```python
from build123d import *

# Parameters (mm, degrees)
F0_W     = 22.098
F0_H     = 47.498
F1_DEPTH = 1016
F2_R     = 3.96875
F3_DEPTH = 1.651
F4_R     = 9.525
F5_DEPTH = 1.651


with BuildPart() as f1:
    # F0 (on Front) → F1 (new body)
    with BuildSketch(Plane.XZ):
        with BuildLine():
            ThreePointArc((0, 1.651), (0.483567, 0.483567), (1.651, 0))
            Line((1.651, 0), (23.749, 0))
            ThreePointArc((23.749, 0), (24.916433, 0.483567), (25.4, 1.651))
            Line((25.4, 1.651), (25.4, 49.149))
            ThreePointArc((25.4, 49.149), (24.916433, 50.316433), (23.749, 50.8))
            Line((23.749, 50.8), (1.651, 50.8))
            ThreePointArc((1.651, 50.8), (0.483567, 50.316433), (0, 49.149))
            Line((0, 49.149), (0, 1.651))
        make_face()
        with Locations((12.7, 25.4)):
            Rectangle(F0_W, F0_H, mode=Mode.SUBTRACT)
    extrude(amount=F1_DEPTH)

    # F2 (on face) → F3 (cut, through all)
    with BuildSketch(Plane.YZ.offset(25.4)):
        with Locations((-508, 25.4)):
            Circle(F2_R)
        with Locations((-53.975, 25.4)):
            Circle(F2_R)
        with Locations((-962.025, 25.4)):
            Circle(F2_R)
    extrude(amount=-F3_DEPTH, mode=Mode.SUBTRACT)

    # F4 (on face) → F5 (cut, through all)
    with BuildSketch(Plane(origin=(0, 0, 0), x_dir=(0, -1, 0), z_dir=(-1, 0, 0))):
        with Locations((508, 25.4)):
            Circle(F4_R)
        with Locations((53.975, 25.4)):
            Circle(F4_R)
        with Locations((962.025, 25.4)):
            Circle(F4_R)
    extrude(amount=-F5_DEPTH, mode=Mode.SUBTRACT)


solid = f1.part
```
The model under review builds one solid part; all positions refer to its coordinate system, in mm. A direction names the side the tool comes from. Give positions to 0.01 mm unless a question says otherwise; leave off trailing zeros. Write each loop counter-clockwise with the first axis right and the second up, starting at its lowest first coordinate (ties: lowest second). Pieces come first, ordered by that corner, then holes. Notation, with made-up numbers: (84.5, 75.25) -> (132.5, 75.25) arc R25 cw to (132.5, 103.25) -> close; hole circle Ø6 at (65.25, 44). An arc over 180 degrees is marked (long way). Answer in a Markdown table with one row per item.
1) Add section B-B on y = -292. State the section outline as (x, z) points.
Worked answers:
| item | result |
|---|---|
| outline | (0, 1.65) arc R1.65 ccw to (1.65, 0) -> (23.75, 0) arc R1.65 ccw to (25.4, 1.65) -> (25.4, 49.15) arc R1.65 ccw to (23.75, 50.8) -> (1.65, 50.8) arc R1.65 ccw to (0, 49.15) -> close; hole (1.65, 1.65) -> (23.75, 1.65) -> (23.75, 49.15) -> (1.65, 49.15) -> close |
2) Clearance check with flat-ended pins moving along their axes: P1, Ø12.5, axis at y = -508, z = 25.4, coming from the -X side; P2, Ø12, axis at x = 13.5, z = 28, coming from the +Y side. State where each tip first meets the part, or that it passes through.
Worked answers:
| item | result |
|---|---|
| P1 | x = 23.75 |
| P2 | through |
3) Tool access review of faces 4 (the flat face through (13, -501, 50.8)), 5 (the cylindrical face through (0.814, -498.484, 25.819)), 6 (the flat face through (13, -501, 1.651)): name each direction out of +Z, -Z, +X, -X, +Y, -Y from which nothing blocks a thin tool from reaching the whole face with its end or side.
Worked answers:
| item | result |
|---|---|
| face 4 | +Z, +X, -X, +Y, -Y |
| face 5 | -X |
| face 6 | +Y, -Y |
4) For L1, parallel to Z at x = 16.5, y = -584; L2, parallel to X at y = -144, z = 6.5; L3, parallel to Z at x = 1.2, y = -508 (3 decimals), list the stretches that pass through material, from the lowest coordinate up. Write a range as [from, to].
Worked answers:
| item | result |
|---|---|
| L1 | [0, 1.65], [49.15, 50.8] |
| L2 | [0, 1.65], [23.75, 25.4] |
| L3 | [0.063, 15.875], [34.925, 50.737] |
5) Add section A-A on x = 14.5. State the section outline as (y, z) points.
Worked answers:
| item | result |
|---|---|
| outline | (-1016, 0) -> (0, 0) -> (0, 1.65) -> (-1016, 1.65) -> close; (-1016, 49.15) -> (0, 49.15) -> (0, 50.8) -> (-1016, 50.8) -> close |
6) Mouldability with a two-part tool opening along Y and no side actions: class faces 1 (the flat face through (1, -1016, 27)), 2 (the flat face through (25.4, -501, 25)), 3 (the cylindrical face through (0.81, -44.46, 25.82)) as +Y half, -Y half, draft (parallel to the pull), parting line (faces both ways), or undercut.
Worked answers:
| item | result |
|---|---|
| face 1 | -Y half |
| face 2 | draft |
| face 3 | undercut |
